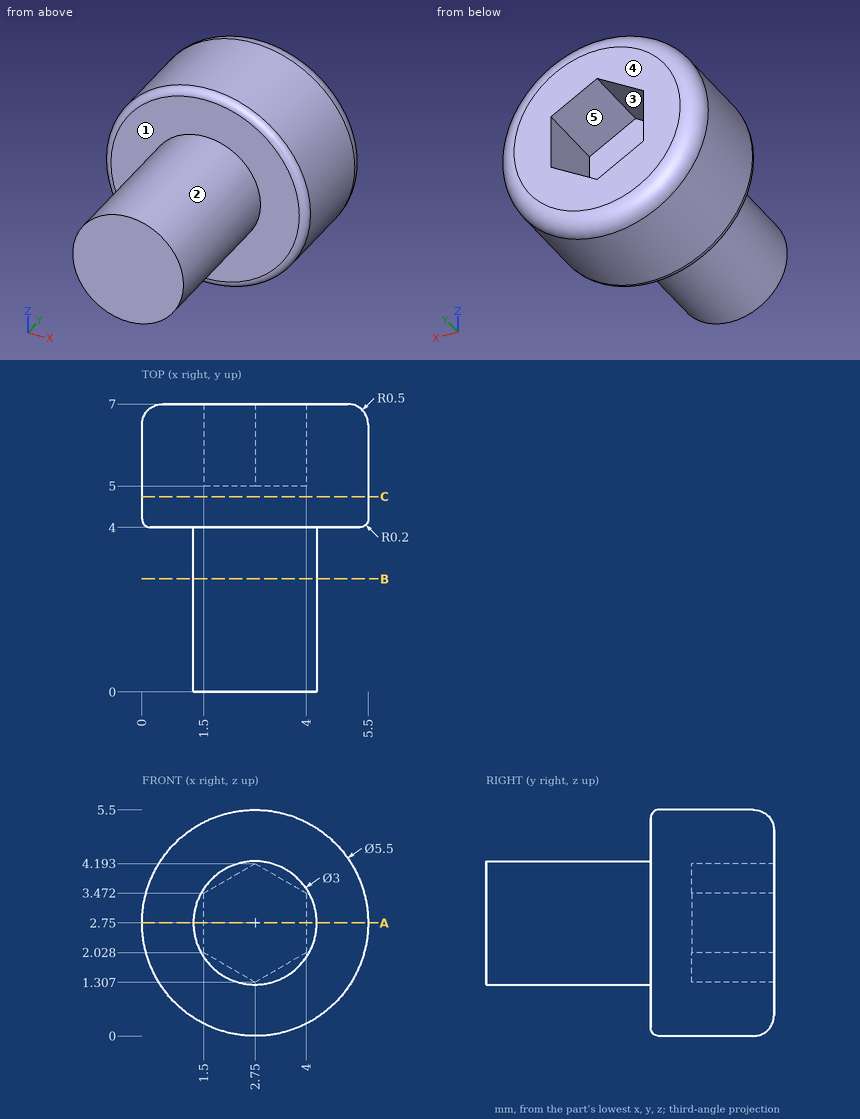
Check sheet for the drawn part. Datum: minimum x, y, z corner. Units: mm. A direction names the side the tool comes from. Round coordinates to 2 decimals unless told otherwise and drop trailing zeros. Write each loop counter-clockwise with the first axis right and the second up, starting at its lowest first coordinate (ties: lowest second). Pieces come first, ordered by that corner, then holes. Notation, with made-up numbers: (-6, 15.5) -> (34, 15.5) arc R24 ccw to (34, 45.5) -> close; hole circle Ø4 at (-29, 5.5). An arc over 180 degrees is marked (long way). Write each question's results on one line, items separated by ' | '. Start each with the question number.
1. Material ranges on probe 1 along Y at (x, z) = (5, 2.55); probe 2 along X at (y, z) = (5.5, 1.8) (1 decimal); probe 3 along Y at (x, z) = (3.8, 2.8), recorded low to high. Write a range as from..to.
2. Cross-section at A-A (z = 2.75). Enter the section's corners in (x, y), then the cut area to 3 significant figures.
3. Cross-section at B-B (y = 2.75). Enter the section's corners in (x, z).
4. Set-up check for the marked faces 4 and 5: record each of +Z, -Z, +X, -X, +Y, -Y from which the full face is reachable in a straight line by a thin tool's end or side.
5. Depth check by flat-ended pin: P1, Ø2, axis at x = 3.5, z = 2, coming from the -Y side. Enter the tip coordinate at first touch or a pass-through.
6. Draft check along Z on the marked faces 1, 2 and 3. Enter one of: +Z half, -Z half, draft (parallel to the pull), parting line (faces both ways), or undercut.
7. Cross-section at C-C (y = 4.75). Enter the section's corners in (x, z).
Solutions:
1) probe 1: y = 4..7 | probe 2: x = 0.2..1.9, 3.6..5.3 | probe 3: y = 0..5
2) outline: (0, 4.2) arc R0.2 ccw to (0.2, 4) -> (1.25, 4) -> (1.25, 0) -> (4.25, 0) -> (4.25, 4) -> (5.3, 4) arc R0.2 ccw to (5.5, 4.2) -> (5.5, 6.5) arc R0.5 ccw to (5, 7) -> (4, 7) -> (4, 5) -> (1.5, 5) -> (1.5, 7) -> (0.5, 7) arc R0.5 ccw to (0, 6.5) -> close | area: 23.4 mm2
3) outline: circle Ø3 at (2.75, 2.75)
4) face 4: +Z, -Z, +X, -X, +Y | face 5: +Y
5) P1: stops at y = 0
6) face 1: draft | face 2: parting line | face 3: undercut
7) outline: circle Ø5.5 at (2.75, 2.75)
